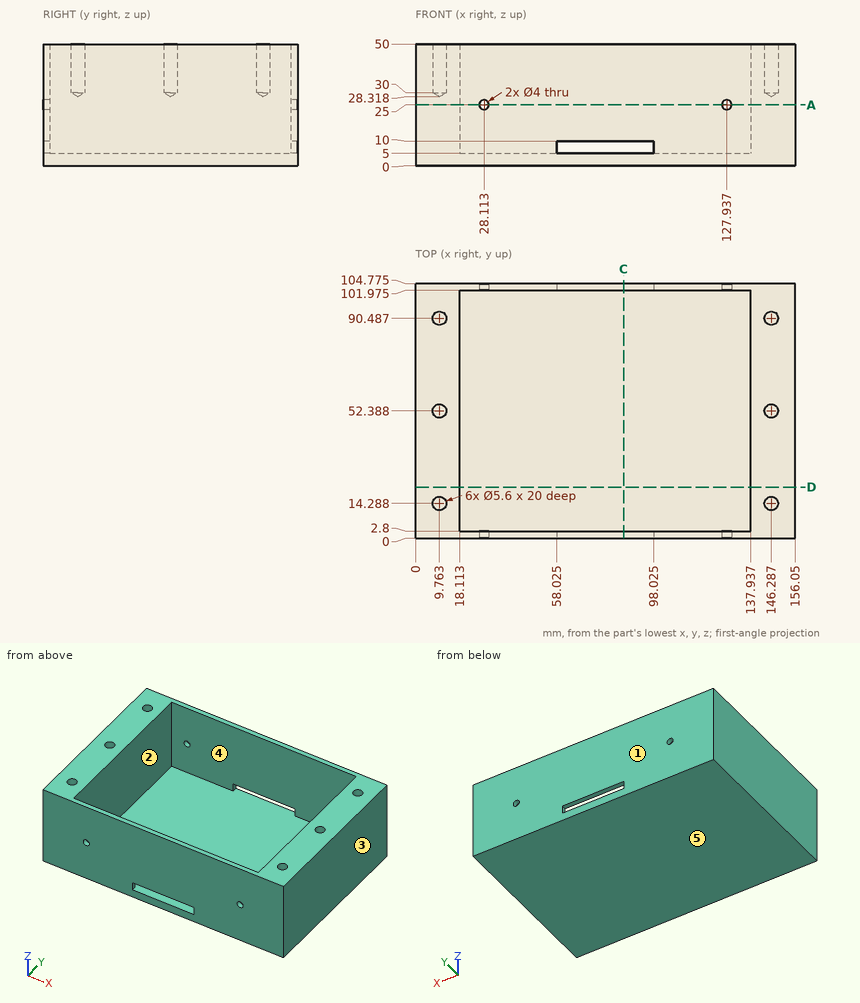
The figure shows three views and two pictorial views of one solid part (mm, origin at its lowest corner). Answer the questions. A direction names the side the tool comes from. Give positions to 0.01 mm unless a question says otherwise; leave off trailing zeros. Order: outer loops, then holes, each group sorted by start corner. A loop starts at its lowest first (then second) coordinate and runs counter-clockwise, first axis right, second up. Notation, with made-up numbers: (23.5, 14) -> (62.5, 14) arc R30 cw to (62.5, 38) -> close; hole circle Ø7 at (48.5, 11). An arc over 180 degrees is marked (long way). Answer as a JSON object with one key per item and string values. Group by question number.
Item 1: The part is cut by section D-D on y = 21. Write down the section's boundary in (x, z).
Item 2: Determine the mould class of the marked faces 3, 4 and 5 for opening direction X: pulls with the +X half, pulls with the -X half, needs draft (parallel to the pull), parting line crosses it, or undercut.
Item 3: A tool of negligible diameter and unlimited length cuts with its end or side. For the marked faces 1 and 2, from which of +Z, -Z, +X, -X, +Y, -Y can it reach the whole face along a straight path? Write none if from no direction.
Item 4: Flat-ended cylindrical pins translate along their axes: pin 1 (6.5 mm diameter, centred on x = 146.287, y = 90.487, fed in from +Z); pin 2 (5 mm diameter, centred on x = 9.763, y = 90.487, fed in from +Z); pin 3 (1.5 mm diameter, centred on x = 47.5, y = 57, fed in from +Z). Find the tip coordinate at first contact, or state that the pin passes through.
Item 5: The part is cut by section C-C on x = 85.5. Write down the section's boundary in (y, z) (1 decimal).
Item 6: Consider L1, parallel to Y at x = 55.5, z = 34 (1 decimal); L2, parallel to X at y = 31, z = 30; L3, parallel to Z at x = 120, y = 83. Determine where each line is inside the solid, lowest interval first. Write a range as from..to.
Item 7: The part is cut by section A-A on z = 25. Give the number of separate pieces and of enclosed holes in the cut face, and give its area (3 significant figures).
Result set:
{
 "1": {"outline": "(0, 0) -> (156.05, 0) -> (156.05, 50) -> (137.94, 50) -> (137.94, 5) -> (18.11, 5) -> (18.11, 50) -> (0, 50) -> close"},
 "2": {"face 3": "pulls with the +X half", "face 4": "undercut", "face 5": "needs draft"},
 "3": {"face 1": "+Z, -Z, +X, -X, +Y", "face 2": "+Z"},
 "4": {"pin 1": "z = 50", "pin 2": "z = 29.82", "pin 3": "z = 5"},
 "5": {"outline": "(0, 0) -> (104.8, 0) -> (104.8, 5) -> (0, 5) -> close; (0, 10) -> (2.8, 10) -> (2.8, 50) -> (0, 50) -> close; (102, 10) -> (104.8, 10) -> (104.8, 50) -> (102, 50) -> close"},
 "6": {"L1": "0..2.8, 102..104.8", "L2": "0..18.11, 137.94..156.05", "L3": "0..5"},
 "7": {"separate pieces": "4", "enclosed holes": "0", "area": "4,420 mm²"}
}
